Work out the finished part from the listing and answer in its coordinate system (mm). Face numbers are marked on the shaded views. Round coordinates to 2 decimals unless told otherwise and drop trailing zeros. Write each loop counter-clockwise with the first axis right and the second up, starting at its lowest first coordinate (ties: lowest second). Pieces come first, ordered by that corner, then holes. Notation, with made-up numbers: (25.25, 61) - (75.25, 61) arc R15 cw to (75.25, 83) - close; hole circle Ø8 at (24.25, -12.75). An arc over 180 degrees is marked (long way). Answer as a JSON object with one key per item and string values.
```python
from build123d import *

# Parameters (mm, degrees)
F0_R     = 35
F0_R_2   = 31.45
F1_DEPTH = 38
F0_R_3   = 29.15
F2_DEPTH = 3.5
F3_R     = 22.2
F4_DEPTH = 25
F5_R     = 25.5
F5_R_2   = 22.2
F6_DEPTH = 35
F7_R     = 29.15
F7_R_2   = 25.5
F8_DEPTH = 35
F9_R     = 5
F10_R    = 5


with BuildPart() as f1:
    # F0 (on Top) → F1 (new body)
    with BuildSketch(Plane.XY):
        Circle(F0_R)
        Circle(F0_R_2, mode=Mode.SUBTRACT)
    extrude(amount=-F1_DEPTH)

    # F0 (on Top) → F2 (join)
    with BuildSketch(Plane.XY):
        Circle(F0_R)
        Circle(F0_R_2, mode=Mode.SUBTRACT)
        Circle(F0_R_2)
        Circle(F0_R_3, mode=Mode.SUBTRACT)
        Circle(F0_R_3)
    extrude(amount=F2_DEPTH)

    # F3 (on face) → F4 (cut)
    with BuildSketch(Plane.XY.offset(3.5)):
        Circle(F3_R)
    extrude(amount=-F4_DEPTH, mode=Mode.SUBTRACT)

    # F5 (on face) → F6 (join)
    with BuildSketch(Plane.XY):
        Circle(F5_R)
        Circle(F5_R_2, mode=Mode.SUBTRACT)
    extrude(amount=-F6_DEPTH)

    # F7 (on face) → F8 (join, through all)
    with BuildSketch(Plane.XY):
        Circle(F7_R)
        Circle(F7_R_2, mode=Mode.SUBTRACT)
    extrude(amount=-F8_DEPTH)

    # F9
    f9_edges = [f1.edges().sort_by_distance(p)[0] for p in [
        (-35, 0, 3.5),
    ]]
    fillet(f9_edges, radius=F9_R)

    # F10
    f10_edges = [f1.edges().sort_by_distance(p)[0] for p in [
        (-29.15, 0, -35),
    ]]
    fillet(f10_edges, radius=F10_R)


solid = f1.part
```
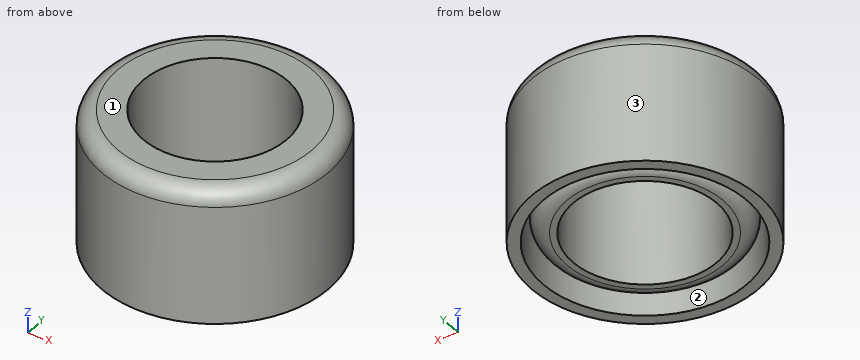
Item 1: Determine the mould class of the marked faces 1, 2 and 3 for opening direction Y: pulls with the +Y half, pulls with the -Y half, needs draft (parallel to the pull), parting line crosses it, or undercut.
Results found:
{"face 1": "needs draft", "face 2": "undercut", "face 3": "parting line crosses it"}
Item 2: Consider line 1 along Y through (x, z) = (0, -12); line 2 along X through (y, z) = (26, -31); line 3 along X through (y, z) = (25, -11.5). Determine where each line is inside the solid, lowest interval first.
Results found:
{"line 1": "-35 to -31.45, -29.15 to -22.2, 22.2 to 29.15, 31.45 to 35", "line 2": "-23.43 to -17.69, -12.96 to 12.96, 17.69 to 23.43", "line 3": "-24.49 to -19.08, -14.99 to 14.99, 19.08 to 24.49"}
Item 3: A cutting plane is placed at C-C (z = -13.5). Write down the section's boundary in (x, y).
Results found:
{"outline": "circle Ø70 at (0, 0); circle Ø58.3 at (0, 0); hole circle Ø62.9 at (0, 0); hole circle Ø44.4 at (0, 0)"}
Item 4: Each of these flat-tipped pins is pushed along its axis until it touches: P1, Ø2, axis at x = 6.5, z = -7, coming from the +Y side; P2, Ø24, axis at x = 3.5, y = -11.5, coming from the -Z side; P3, Ø8, axis at y = -5, z = -3, coming from the +X side. Where does it stop, or does it pass through?
Results found:
{"P1": "y = 34.57", "P2": "z = -35", "P3": "x = 34.99"}
Item 5: A cutting plane is placed at A-A (y = 0). Write down the section's boundary in (x, z).
Results found:
{"outline": "(-35, -38) - (-31.45, -38) - (-31.45, 0) - (-29.15, 0) - (-29.15, -30) arc R5 ccw to (-24.15, -35) - (-22.2, -35) - (-22.2, 3.5) - (-30, 3.5) arc R5 ccw to (-35, -1.5) - close; (22.2, -35) - (24.15, -35) arc R5 ccw to (29.15, -30) - (29.15, 0) - (31.45, 0) - (31.45, -38) - (35, -38) - (35, -1.5) arc R5 ccw to (30, 3.5) - (22.2, 3.5) - close"}
